For this review, use the dimensioned drawing (mm, ordinates from the lowest corner) and the shaded views. Give positions to 0.01 mm unless a question says otherwise; leave off trailing zeros. Loops run counter-clockwise (first coordinate to the right, second up) from the corner with the lowest first, then second, coordinate; pieces in that order, holes last. Notation, with made-up numbers: M -28,-16 L 7,-16 A25 ccw 7,18 Z; hole C 29.5,12.5 d11. An arc over 180 degrees is marked long. Use a Markdown table: item, result. Add a question column.
(1) Add section C-C, the plane x = 76. Give the boundary of the cut face in (y, z) (1 decimal).
(2) Insertion check: pin 1 Ø12 at (y, z) = (95.5, 11.5) entering from -X; pin 2 Ø5 at (y, z) = (87, 3) entering from +X (1 decimal); pin 3 Ø2 at (y, z) = (20, 6.5) entering from +X. Each pin has a flat end and moves straight along its axis. Give the tip position at first contact, or say it passes through.
(3) Add section A-A, the plane x = 24.5. Give the boundary of the cut face in (y, z), then the cut area to 3 significant figures.
(4) For probe 1 along X at (y, z) = (39.5, 19.75) (1 decimal); probe 2 along Y at (x, z) = (52.5, 3) (1 decimal); probe 3 along X at (y, z) = (41.5, 17.25) (1 decimal), list the stretches that pass through material, from the lowest coordinate up.
(5) Add section D-D, the plane z = 14.75. State how many separate pieces and enclosed holes the cut face has, then the cut area to 3 significant figures.
(6) Add section B-B, the plane y = 66. Give the boundary of the cut face in (x, z), then the cut area to 4 significant figures.
(7) Draft analysis for pull direction Y (two halves, no side actions). For the marked faces 1, 2, 3 and 4, state which applies: pulls with the +Y half, pulls with the -Y half, needs draft (parallel to the pull), parting line crosses it, or undercut.
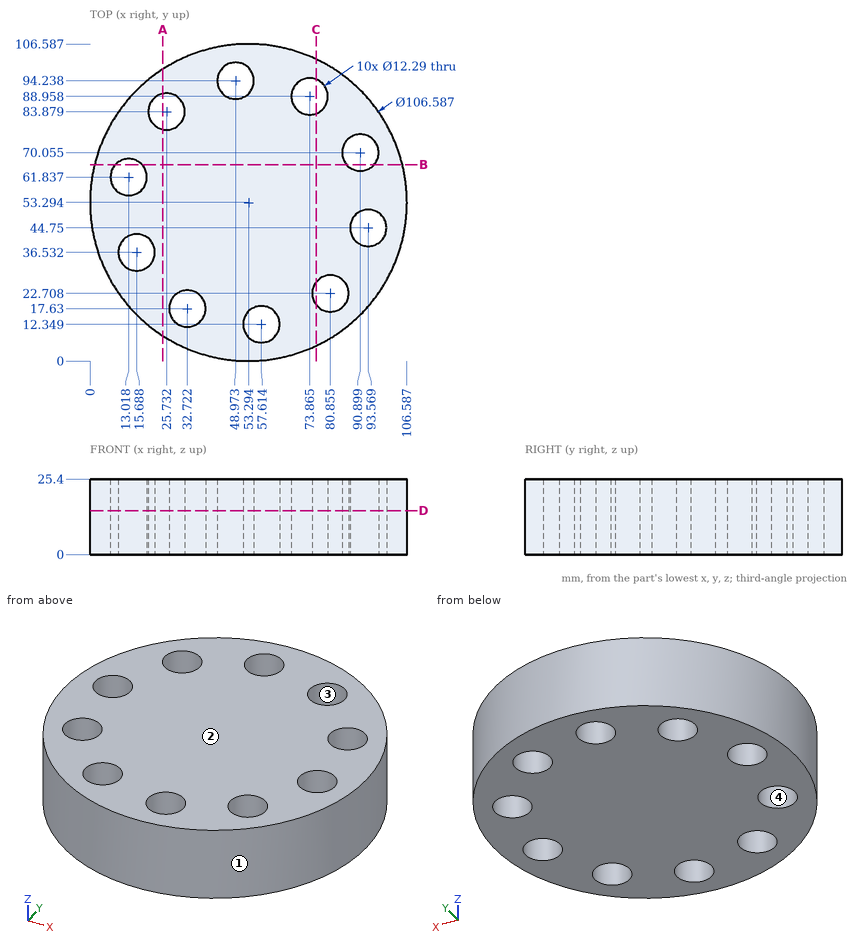
Established:
| question | item | result |
|---|---|---|
| 1 | outline | M 5.1,0 L 18.9,0 L 18.9,25.4 L 5.1,25.4 Z; M 26.5,0 L 83.2,0 L 83.2,25.4 L 26.5,25.4 Z; M 94.7,0 L 101.5,0 L 101.5,25.4 L 94.7,25.4 Z |
| 2 | pin 1 | x = 14.19 |
| 2 | pin 2 | x = 96.5 |
| 2 | pin 3 | x = 95.69 |
| 3 | outline | M 8.45,0 L 77.86,0 L 77.86,25.4 L 8.45,25.4 Z; M 89.9,0 L 98.14,0 L 98.14,25.4 L 89.9,25.4 Z |
| 3 | area | 1,970 mm^2 |
| 4 | probe 1 | 1.8 to 10.3, 21.1 to 90.4, 96.8 to 104.8 |
| 4 | probe 2 | 0 to 8.9, 15.8 to 89.2, 99.3 to 106.6 |
| 4 | probe 3 | 1.3 to 12.1, 19.3 to 88.4, 98.8 to 105.3 |
| 5 | separate pieces | 1 |
| 5 | enclosed holes | 10 |
| 5 | area | 7,740 mm^2 |
| 6 | outline | M 1.54,0 L 8.5,0 L 8.5,25.4 L 1.54,25.4 Z; M 17.54,0 L 86.28,0 L 86.28,25.4 L 17.54,25.4 Z; M 95.52,0 L 105.05,0 L 105.05,25.4 L 95.52,25.4 Z |
| 6 | area | 2,165 mm^2 |
| 7 | face 1 | parting line crosses it |
| 7 | face 2 | needs draft |
| 7 | face 3 | undercut |
| 7 | face 4 | undercut |
